```python
from build123d import *

# Parameters (mm, degrees)
F0_R      = 4
F1_DEPTH  = 7
F2_SIZE   = 0.5
F3_R      = 6
F4_DEPTH  = 391
F5_R      = 4
F6_DEPTH  = 12
F7_SIZE   = 0.5
F8_R      = 2.5
F9_DEPTH  = 10
F10_SIZE  = 0.5
F12_DEPTH = 7


with BuildPart() as f1:
    # F0 (on Top) → F1 (new body)
    with BuildSketch(Plane.XY):
        Circle(F0_R)
    extrude(amount=-F1_DEPTH)

    # F2
    f2_edges = [f1.edges().sort_by_distance(p)[0] for p in [
        (-4, 0, 0),
    ]]
    chamfer(f2_edges, length=F2_SIZE)

    # F3 (on face) → F4 (join)
    with BuildSketch(Plane(origin=(0, 0, -7), x_dir=(1, 0, 0), z_dir=(0, 0, -1))):
        Circle(F3_R)
    extrude(amount=F4_DEPTH)

    # F5 (on face) → F6 (join)
    with BuildSketch(Plane(origin=(0, 0, -398), x_dir=(1, 0, 0), z_dir=(0, 0, -1))):
        Circle(F5_R)
    extrude(amount=F6_DEPTH)

    # F7
    f7_edges = [f1.edges().sort_by_distance(p)[0] for p in [
        (-4, 0, -410),
    ]]
    chamfer(f7_edges, length=F7_SIZE)

    # F8 (on face) → F9 (join)
    with BuildSketch(Plane(origin=(0, 0, -410), x_dir=(1, 0, 0), z_dir=(0, 0, -1))):
        Circle(F8_R)
    extrude(amount=F9_DEPTH)

    # F10
    f10_edges = [f1.edges().sort_by_distance(p)[0] for p in [
        (-2.5, 0, -420),
    ]]
    chamfer(f10_edges, length=F10_SIZE)

    # F11 (on face) → F12 (cut)
    with BuildSketch(Plane(origin=(0, 0, -420), x_dir=(1, 0, 0), z_dir=(0, 0, -1))):
        with BuildLine():
            Line((1.3228756555, -1.5), (-1.3228756555, -1.5))
            ThreePointArc((-1.3228756555, -1.5), (0, -2), (1.3228756555, -1.5))
        make_face()
        with BuildLine():
            Line((-1.3228756555, -1.5), (-2, -1.5))
            ThreePointArc((-2, -1.5), (0, -2.5), (2, -1.5))
            Line((2, -1.5), (1.3228756555, -1.5))
            ThreePointArc((1.3228756555, -1.5), (0, -2), (-1.3228756555, -1.5))
        make_face()
    extrude(amount=-F12_DEPTH, mode=Mode.SUBTRACT)


solid = f1.part
```
Part model, mm, in its own coordinate system. A direction names the side the tool comes from. Coordinates: 2 decimals unless noted, no trailing zeros. Loops run counter-clockwise (first coordinate to the right, second up) from the corner with the lowest first, then second, coordinate; pieces in that order, holes last. Notation, with made-up numbers: (77.25, 83.5) - (87.25, 83.5) arc R13 ccw to (87.25, 103.5) - close; hole circle Ø10 at (12.25, -28.5). An arc over 180 degrees is marked (long way). Write item = value, one per line. Start each with the question number.
Item 1: 3-axis set-ups, long thin cutter, end or side, ignore diameter. For faces 1 (the flat face through (-1.42, 3.92, -398)), 2 (the cylindrical face through (-0.867, -3.905, -3.704)), 3 (the flat face through (0, 0, 0)): which of +Z, -Z, +X, -X, +Y, -Y reach the whole face in a straight line?
Item 2: Cut at A-A, the plane z = -113.5. Give the cut face in (x, y), and give its area (3 significant figures).
Item 3: Wall check: L1, parallel to Z at x = 0.5, y = 2; L2, parallel to Z at x = 5, y = 0; L3, parallel to Y at x = 1, z = -374.5. Give the ranges that are in metal, low to high. Write a range as from..to.
Item 4: Flat gauge pins, fed straight in: pin 1 Ø1 at (y, z) = (-4.5, -236.5) entering from +X; pin 2 Ø1 at (x, z) = (3, -162.5) entering from +Y; pin 3 Ø2 at (y, z) = (-3.5, -83) entering from -X. Where does each tip first touch, or does it go through?
The answers:
q1.face_1 = -Z
q1.face_2 = +Z
q1.face_3 = +Z, +X, -X, +Y, -Y
q2.outline = circle Ø12 at (0, 0)
q2.area = 113 mm2
q3.L1 = -413..0
q3.L2 = -398..-7
q3.L3 = -5.92..5.92
q4.pin_1 = 4.47
q4.pin_2 = 5.45
q4.pin_3 = -5.45
